Build history of the part. All positions in model axes, mm. A direction names the side the tool comes from. Round coordinates to 2 decimals unless told otherwise and drop trailing zeros. Write each loop counter-clockwise with the first axis right and the second up, starting at its lowest first coordinate (ties: lowest second). Pieces come first, ordered by that corner, then holes.
from build123d import *

# Parameters (mm, degrees)
BOSS_EXTRUDE1_DEPTH     = 12.7
BACKREST_BRACKET_SLOT_W = 12.7
BACKREST_BRACKET_SLOT_H = 8.89
CUT_EXTRUDE3_DEPTH      = 12.7
BACKREST_SCREW_HOLE_R   = 1.397
CUT_EXTRUDE4_DEPTH      = 6.35
CUT_EXTRUDE5_DEPTH      = 25.4
BOSS_EXTRUDE2_DEPTH     = 3.175
SKETCH37_W              = 12.7
SKETCH37_H              = 101.6
CUT_EXTRUDE7_DEPTH      = 8.89
SKETCH38_R              = 3.175
CUT_EXTRUDE8_DEPTH      = 12.7


with BuildPart() as part:
    # Main Body → Boss-Extrude1 (new body)
    with BuildSketch(Plane(origin=(0, 0, 0), x_dir=(1, 0, 0), z_dir=(0, 1, 0))):
        with BuildLine():
            Line((-301.625, -95.25), (-301.625, 95.25))
            ThreePointArc((-301.625, 95.25), (-296.045384182, 108.720384182), (-282.575, 114.3))
            Line((-282.575, 114.3), (282.575, 114.3))
            ThreePointArc((282.575, 114.3), (296.045384182, 108.720384182), (301.625, 95.25))
            Line((301.625, 95.25), (301.625, -95.25))
            ThreePointArc((301.625, -95.25), (296.045384182, -108.720384182), (282.575, -114.3))
            Line((282.575, -114.3), (-282.575, -114.3))
            ThreePointArc((-282.575, -114.3), (-296.045384182, -108.720384182), (-301.625, -95.25))
        make_face()
    extrude(amount=BOSS_EXTRUDE1_DEPTH)

    # Backrest Bracket Slot → Cut-Extrude3 (cut)
    with BuildSketch(Plane.XY.offset(114.3)):
        with Locations((-276.225, 8.255)):
            Rectangle(BACKREST_BRACKET_SLOT_W, BACKREST_BRACKET_SLOT_H)
    cut_extrude3 = extrude(amount=-CUT_EXTRUDE3_DEPTH, mode=Mode.SUBTRACT)

    # Backrest Screw Hole → Cut-Extrude4 (cut)
    with BuildSketch(Plane.XY.offset(101.6)):
        with Locations((-276.225, 8.255)):
            Circle(BACKREST_SCREW_HOLE_R)
    cut_extrude4 = extrude(amount=-CUT_EXTRUDE4_DEPTH, mode=Mode.SUBTRACT)

    # Mirror1: Cut-Extrude3, Cut-Extrude4 across plane
    add(cut_extrude3.mirror(Plane.XY), mode=Mode.SUBTRACT)
    add(cut_extrude4.mirror(Plane.XY), mode=Mode.SUBTRACT)

    # Couch Foot Slits → Cut-Extrude5 (cut)
    with BuildSketch(Plane(origin=(0, 12.7, 0), x_dir=(1, 0, 0), z_dir=(0, 1, 0))):
        with BuildLine():
            Line((-231.775, 88.9), (-168.275, 88.9))
            Line((-168.275, 88.9), (-168.275, 50.8))
            Line((-168.275, 50.8), (-231.775, 50.8))
            ThreePointArc((-231.775, 50.8), (-240.755256121, 54.519743879), (-244.475, 63.5))
            Line((-244.475, 63.5), (-244.475, 76.2))
            ThreePointArc((-244.475, 76.2), (-240.755256121, 85.180256121), (-231.775, 88.9))
        make_face()
        with BuildLine():
            Line((276.225, 76.2), (276.225, 63.5))
            ThreePointArc((276.225, 63.5), (272.505256121, 54.519743879), (263.525, 50.8))
            Line((263.525, 50.8), (200.025, 50.8))
            Line((200.025, 50.8), (200.025, 88.9))
            Line((200.025, 88.9), (263.525, 88.9))
            ThreePointArc((263.525, 88.9), (272.505256121, 85.180256121), (276.225, 76.2))
        make_face()
        with BuildLine():
            Line((-231.775, -50.8), (-168.275, -50.8))
            Line((-168.275, -50.8), (-168.275, -88.9))
            Line((-168.275, -88.9), (-231.775, -88.9))
            ThreePointArc((-231.775, -88.9), (-240.755256121, -85.180256121), (-244.475, -76.2))
            Line((-244.475, -76.2), (-244.475, -63.5))
            ThreePointArc((-244.475, -63.5), (-240.755256121, -54.519743879), (-231.775, -50.8))
        make_face()
        with BuildLine():
            Line((276.225, -63.5), (276.225, -76.2))
            ThreePointArc((276.225, -76.2), (272.505256121, -85.180256121), (263.525, -88.9))
            Line((263.525, -88.9), (200.025, -88.9))
            Line((200.025, -88.9), (200.025, -50.8))
            Line((200.025, -50.8), (263.525, -50.8))
            ThreePointArc((263.525, -50.8), (272.505256121, -54.519743879), (276.225, -63.5))
        make_face()
    extrude(amount=-CUT_EXTRUDE5_DEPTH, mode=Mode.SUBTRACT)

    # Sketch24 → Boss-Extrude2 (add, symmetric)
    with BuildSketch(Plane(origin=(0, 6.35, 0), x_dir=(1, 0, 0), z_dir=(0, 1, 0))):
        with BuildLine():
            Line((0.635, -120.65), (26.035, -120.65))
            ThreePointArc((26.035, -120.65), (30.525128061, -118.790128061), (32.385, -114.3))
            Line((32.385, -114.3), (34.925, -114.3))
            ThreePointArc((34.925, -114.3), (32.321179285, -120.586179285), (26.035, -123.19))
            Line((26.035, -123.19), (0.635, -123.19))
            ThreePointArc((0.635, -123.19), (-5.651179285, -120.586179285), (-8.255, -114.3))
            Line((-8.255, -114.3), (-5.715, -114.3))
            ThreePointArc((-5.715, -114.3), (-3.855128061, -118.790128061), (0.635, -120.65))
        make_face()
        with BuildLine():
            Line((-241.935, -120.65), (-216.535, -120.65))
            ThreePointArc((-216.535, -120.65), (-212.044871939, -118.790128061), (-210.185, -114.3))
            Line((-210.185, -114.3), (-207.645, -114.3))
            ThreePointArc((-207.645, -114.3), (-210.248820715, -120.586179285), (-216.535, -123.19))
            Line((-216.535, -123.19), (-241.935, -123.19))
            ThreePointArc((-241.935, -123.19), (-248.221179285, -120.586179285), (-250.825, -114.3))
            Line((-250.825, -114.3), (-248.285, -114.3))
            ThreePointArc((-248.285, -114.3), (-246.425128061, -118.790128061), (-241.935, -120.65))
        make_face()
        with BuildLine():
            Line((243.205, -120.65), (268.605, -120.65))
            ThreePointArc((268.605, -120.65), (273.095128061, -118.790128061), (274.955, -114.3))
            Line((274.955, -114.3), (277.495, -114.3))
            ThreePointArc((277.495, -114.3), (274.891179285, -120.586179285), (268.605, -123.19))
            Line((268.605, -123.19), (243.205, -123.19))
            ThreePointArc((243.205, -123.19), (236.918820715, -120.586179285), (234.315, -114.3))
            Line((234.315, -114.3), (236.855, -114.3))
            ThreePointArc((236.855, -114.3), (238.714871939, -118.790128061), (243.205, -120.65))
        make_face()
    boss_extrude2 = extrude(amount=BOSS_EXTRUDE2_DEPTH, both=True)

    # Mirror2: Boss-Extrude2 across plane
    add(boss_extrude2.mirror(Plane.XY))

    # Sketch37 → Cut-Extrude7 (cut)
    with BuildSketch(Plane(origin=(0, 12.7, 0), x_dir=(1, 0, 0), z_dir=(0, 1, 0))):
        with Locations((-276.225, 0)):
            Rectangle(SKETCH37_W, SKETCH37_H)
    extrude(amount=-CUT_EXTRUDE7_DEPTH, mode=Mode.SUBTRACT)

    # Sketch38 → Cut-Extrude8 (cut)
    with BuildSketch(Plane(origin=(0, 12.7, 0), x_dir=(1, 0, 0), z_dir=(0, 1, 0))):
        with Locations((-229.235, -101.6)):
            Circle(SKETCH38_R)
        with Locations((13.335, -101.6)):
            Circle(SKETCH38_R)
        with Locations((255.905, -101.6)):
            Circle(SKETCH38_R)
    cut_extrude8 = extrude(amount=-CUT_EXTRUDE8_DEPTH, mode=Mode.SUBTRACT)

    # Mirror3: Cut-Extrude8 across plane
    add(cut_extrude8.mirror(Plane.XY), mode=Mode.SUBTRACT)


solid = part.part
1) Which spindle directions (+Z, -Z, +X, -X, +Y, -Y) get a long thin tool onto all of the face, cutting with end or side? Do faces 1 (the cylindrical face through (-295.896, 6.261, 108.868)), 2 (the flat face through (-168.275, 6, 70)). Say none if no direction does.
Results:
face 1: +Z, -X, +Y, -Y
face 2: +Y, -Y
2) Mould opens along Z. For faces 3 (the flat face through (4, 12.7, -2)), 4 (the cylindrical face through (296.193, 6.261, 108.571)), 5 (the flat face through (-200, 6, -50.8)) say: released by +Z, released by -Z, zero draft, split by the parting line, or undercut.
Results:
face 3: zero draft
face 4: released by +Z
face 5: undercut
3) Pin check, flat tips, straight feed: pin 1 Ø6.5 at (x, y) = (-193, 6.5) entering from -Z; pin 2 Ø4.5 at (y, z) = (10, 111) entering from +X; pin 3 Ø6.5 at (x, y) = (239.5, 4) entering from +Z. Stop position of each tip, or through.
Results:
pin 1: stops at z = -114.3
pin 2: stops at x = 296.02
pin 3: stops at z = 123.18
4) Slice it at A-A (x = -201.5). Write the cut outline in (y, z).
Results:
outline: (0, -114.3) - (12.7, -114.3) - (12.7, -88.9) - (0, -88.9) - close; (0, -50.8) - (12.7, -50.8) - (12.7, 50.8) - (0, 50.8) - close; (0, 88.9) - (12.7, 88.9) - (12.7, 114.3) - (0, 114.3) - close
5) Slice it at B-B (x = 174). Write the cut outline in (y, z).
Results:
outline: (0, -114.3) - (12.7, -114.3) - (12.7, 114.3) - (0, 114.3) - close
6) Wall check: L1, parallel to Z at x = 14, y = 6.5; L2, parallel to Z at x = 249.5, y = 7.25; L3, parallel to Z at x = -202.5, y = 7.25. Give the ranges that are in metal, low to high.
Results:
L1: z = -123.19 to -120.65, -114.3 to -104.7, -98.5 to 98.5, 104.7 to 114.3, 120.65 to 123.19
L2: z = -123.19 to -120.65, -114.3 to -88.9, -50.8 to 50.8, 88.9 to 114.3, 120.65 to 123.19
L3: z = -114.3 to -88.9, -50.8 to 50.8, 88.9 to 114.3
